```python
from build123d import *

# Parameters (mm, degrees)
BOSS_EXTRUDE1_DEPTH = 2.54
SKETCH1_4_R         = 1.27
CUT_EXTRUDE1_DEPTH  = 3.302


with BuildPart() as part:
    # Sketch1 → Boss-Extrude1 (new body)
    with BuildSketch(Plane.XY):
        Polygon((-67.806668191, 8.452347061), (-29.139739371, 35.905866523), (-24.728354348, 29.69264818), (-63.395283168, 2.239128718), align=None)
    extrude(amount=BOSS_EXTRUDE1_DEPTH)

    # Sketch1<4> → Cut-Extrude1 (cut)
    with BuildSketch(Plane.XY):
        with Locations((-62.437432462, 7.591853574)):
            Circle(SKETCH1_4_R)
        with Locations((-30.019544177, 30.608554257)):
            Circle(SKETCH1_4_R)
    extrude(amount=CUT_EXTRUDE1_DEPTH, mode=Mode.SUBTRACT)


solid = part.part
```
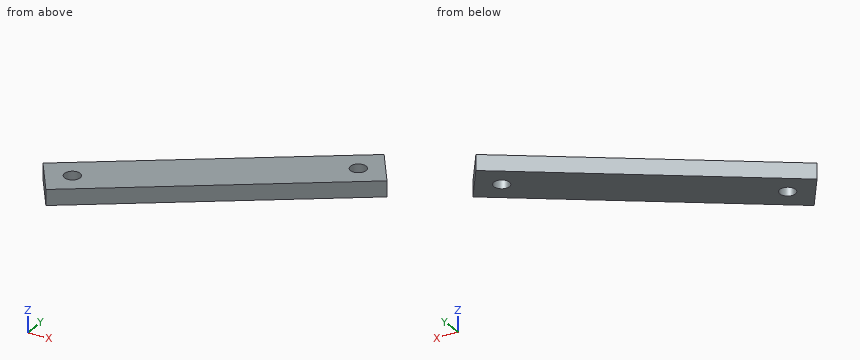
The listing builds one solid part. Answer for the finished solid, in the listing's coordinates (mm). Coordinates: 2 decimals unless noted, no trailing zeros. Write each loop counter-clockwise with the first axis right and the second up, starting at its lowest first coordinate (ties: lowest second). Pieces come first, ordered by that corner, then holes. Notation, with made-up numbers: (-19, 12.5) - (3, 12.5) arc R21 ccw to (3, 16.5) - close; hole circle Ø7 at (46.25, -14). An arc over 180 degrees is marked (long way). Return JSON: item names as keys, results as strings. Group by question number.
1. Straight lines are drawn through the part: L1, parallel to Y at x = -61.5, z = 0.2; L2, parallel to X at y = 29, z = 1.5; L3, parallel to Y at x = -49, z = 0.45. For each, find the intervals that lie inside material, in ascending order.
2. A cutting plane is placed at A-A, the plane z = 1.25. Determine the outline of the cut face in (x, y), plus the area to 3 significant figures.
3. A cutting plane is placed at C-C, the plane x = -60. Determine the outline of the cut face in (y, z), plus the area to 3 significant figures.
4. A cutting plane is placed at B-B, the plane y = 26. Determine the outline of the cut face in (x, z).
5. Given pin 1 (1.5 mm diameter, centred on x = -43, z = 1, fed in from -Y); pin 2 (1.5 mm diameter, centred on y = 7.5, z = 2, fed in from +X); pin 3 (1.5 mm diameter, centred on x = -34.5, z = 1, fed in from -Y), each flat-ended and moving along its own axis, determine where each tip first touches the part or whether it passes through.
Ans:
{
 "1": {"L1": "3.58 to 6.74, 8.45 to 12.93", "L2": "-38.87 to -25.7", "L3": "12.46 to 21.81"},
 "2": {"outline": "(-67.81, 8.45) - (-63.4, 2.24) - (-24.73, 29.69) - (-29.14, 35.91) - close; hole circle Ø2.54 at (-62.44, 7.59); hole circle Ø2.54 at (-30.02, 30.61)", "area": "351 mm²"},
 "3": {"outline": "(4.65, 0) - (14, 0) - (14, 2.54) - (4.65, 2.54) - close", "area": "23.7 mm²"},
 "4": {"outline": "(-43.09, 0) - (-29.93, 0) - (-29.93, 2.54) - (-43.09, 2.54) - close"},
 "5": {"pin 1": "y = 16.19", "pin 2": "x = -54.93", "pin 3": "y = 22.22"}
}
